Autodesk Inventor part; units mm, degrees
ref_plane "Work Plane1" through (30, 0, 0) normal (0, -0.5, 0.866) x (1, 0, 0)
ref_plane "YZ Plane" through (0, 0, 0) normal (1, 0, 0) x (0, 1, 0)
ref_plane "XZ Plane" through (0, 0, 0) normal (0, 1, 0) x (-1, 0, 0)
sketch "Sketch1" plane through (0, 0, 0) normal (0, 0, 1) x (1, 0, 0)
  line L0 (-0.6667, 0) -> (12, 0)
  line L1 (12, 0) -> (12, 1.5)
  line L2 (12, 1.5) -> (1.3067, 1.5)
  line L3 (1.3067, 1.5) -> (1, 1.5)
  line L4 (1, 1.5) -> (0, 1.5)
  line L5 (0, 1.5) -> (0, 2.75)
  line L6 (0, 2.75) -> (-3, 2.75)
  line L7 (-3, 2.75) -> (-3, 1.4434)
  line L8 (-3, 1.4434) -> (-1.5, 1.4434)
  line L9 (-1.5, 1.4434) -> (-0.6667, 0)
  line L10 (-6, 0) -> (15, 0)
  line L11 (0, -0.55) -> (0, 3.3)
  line L12 (1.3067, 1.5) -> (0, 1.5) construction
  dimension "d0" = 10.6933
  dimension "d1" = 0.3067
  dimension "d2" = 3
  dimension "d3" = 1.5
  dimension "d4" = 60
  dimension "d5" = 3
  dimension "d6" = 3
  dimension "d7" = 2.8868
  dimension "d8" = 5.5
  dimension "d19" = 12
revolve "Body" add sketch "Sketch1" angle 360 about axis through (-0.6667, 0, 0) along (1, 0, 0)
sketch "Sketch2" plane through (-3, 0, 0) normal (-1, 0, 0) x (0, 0, 1)
  circle A0 centre (0, 0) radius 1.4434
  line L0 (0, -3.85) -> (0, 3.85)
  line L1 (-3.85, 0) -> (3.85, 0)
  line L2 (1.4434, 0) -> (0.7217, -1.25)
  line L3 (0.7217, -1.25) -> (-0.7217, -1.25)
  line L4 (-0.7217, -1.25) -> (-1.4434, 0)
  line L5 (-1.4434, 0) -> (-0.7217, 1.25)
  line L6 (-0.7217, 1.25) -> (0.7217, 1.25)
  line L7 (0.7217, 1.25) -> (1.4434, 0)
  point P0 (0, 0)
extrude "Slot" add sketch "Sketch2" against normal up to next contours L7 A0 | A0 L2 | L6 L0 A0 | A0 L0 L3 | L0 L6 A0 | A0 L3 L0 | L4 A0 | A0 L5
fillet "Fillet2" radius 0.3 1 edges at (-3, -2.75, 0)
thread "Thread"
chamfer "Chamfer1" distance 0.3067 distance2 0.3067 1 edges at (12, -1.5, 0) measured on face at (12, -0.6587, -0.1791)
fillet "Fillet1" radius 0.1 1 edges at (0, -1.5, 0)
ref_plane "Work Plane1" through (30, 0, 0) normal (0, -0.5, 0.866) x (1, 0, 0)
equation "\"d0\" = GEL"
equation "\"d1\" = GAL"
equation "\"d2\" = KOH"
equation "\"d3\" = INTI"
equation "\"d5\" = GD"
equation "\"d6\" = BDM"
equation "\"d7\" = 1.1547 * SW"
equation "\"d8\" = KOD"
equation "\"d19\" = NLG"
equation "\"d16\" = RR"
equation "\"d12\" = GEL"
equation "\"d14\" = -0.5 * SPD + 0.5 * GD"
equation "\"d15\" = GUL"
equation "\"d29\" = R"
equation "\"GD\" = NND"
equation "\"NLG\" = 12"
equation "\"GEL\" = 10.69327"
equation "\"KOD\" = 5.5"
equation "\"KOH\" = 3"
equation "\"INTI\" = 1.5"
equation "\"GAL\" = 0.61345 * PTC"
equation "\"GUL\" = 0.61345 * PTC"
equation "\"BDM\" = NND"
equation "\"SW\" = 2.5"
equation "\"RR\" = 0.3"
equation "\"SPD\" = 2.38655"
equation "\"d28\" = R"
equation "\"R\" = 0.1"
equation "\"TOA\" = 30deg"
equation "\"THREADDIA\" = 3"
equation "\"KOD1\" = KOD"
equation "\"PTC\" = 0.5"
equation "\"NND\" = 3"
equation "\"E0\" = 1.155 * SW"
equation "\"GD1\" = THREADDIA - 1.2269 * PTC"
properties part number "ANSI B18.3.1M - M3x0.5 x 12" material "Steel, Mild"
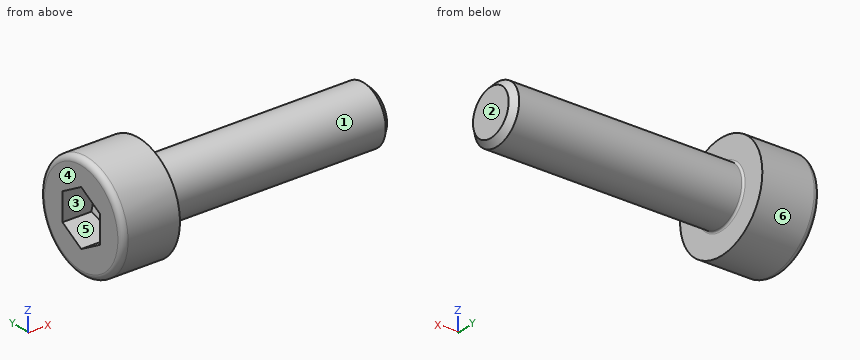
Geometry: final body of the model. Coordinates: model frame, mm. Face numbers are marked on the shaded views. A direction names the side the tool comes from. Give positions to 0.01 mm unless a question says otherwise; leave off trailing zeros. Write each loop counter-clockwise with the first axis right and the second up, starting at its lowest first coordinate (ties: lowest second). Pieces come first, ordered by that corner, then holes. Notation, with made-up numbers: (35, 50.25) - (89, 50.25) arc R6 cw to (89, 56.25) - close; hole circle Ø9 at (13, -24). An arc over 180 degrees is marked (long way). Return JSON: item names as keys, results as strings. Group by question number.
1) Line query: line 1 (X direction, y = 0.65, z = 2); line 2 (Y direction, x = 4, z = 0.1); line 3 (Z direction, x = -1.5, y = 0.9). Output: solid intervals per line, ascending.
2) Mould query, pull axis Z, two halves, no side actions, for the marked faces 4, 5 and 6. Classes: released by +Z, released by -Z, zero draft, split by the parting line, or undercut.
3) Set-up query: the marked faces 1, 2 and 3. Return all of +Z, -Z, +X, -X, +Y, -Y with unobstructed straight access to the full face (end or side cutting, diameter ignored); none if empty.
4) Section A-A on x = 5.5. Return the cut outline in (y, z).
5) First-contact query: P1, Ø1.5, axis at x = 3.5, y = 0, coming from the +Z side; P2, Ø1.5, axis at x = 0, z = -2, coming from the -Y side; P3, Ø2, axis at x = 6, z = -1, coming from the +Y side. Flat tips, straight axial feed; report the tip coordinate or a pass-through.
Filled in:
{
 "1": {"line 1": "x = -3 to 0", "line 2": "y = -1.5 to 1.5", "line 3": "z = -2.6 to -0.92, 0.92 to 2.6"},
 "2": {"face 4": "zero draft", "face 5": "undercut", "face 6": "split by the parting line"},
 "3": {"face 1": "+X", "face 2": "+Z, -Z, +X, +Y, -Y", "face 3": "-X"},
 "4": {"outline": "circle Ø3 at (0, 0)"},
 "5": {"P1": "stops at z = 1.5", "P2": "stops at y = -2.45", "P3": "stops at y = 1.5"}
}
